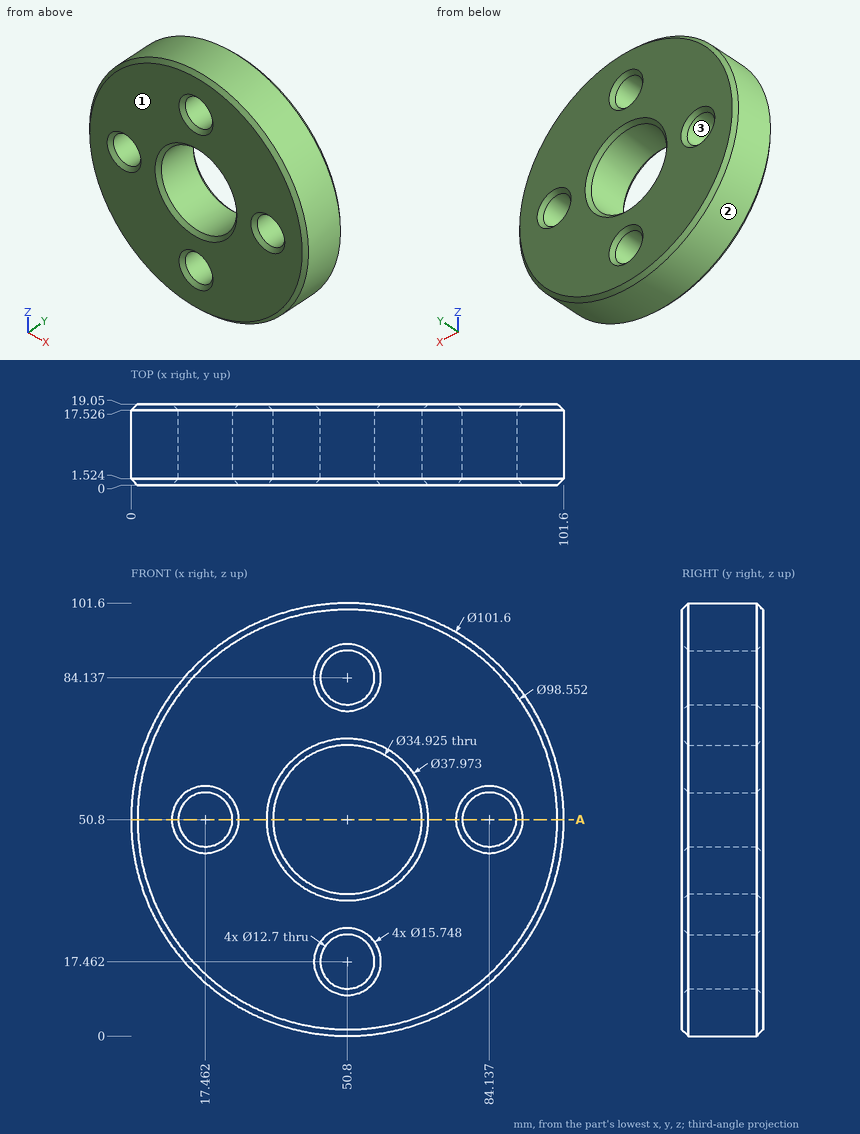
Job drawing, mm, ordinate dimensions from the low corner. One solid piece. Round coordinates to 2 decimals unless told otherwise and drop trailing zeros.
Item 1: Drop flat-ended pins along their axis: P1, Ø10, axis at x = 84.14, z = 50.8, coming from the +Y side; P2, Ø2, axis at x = 26.5, y = 12.5, coming from the -Z side; P3, Ø6, axis at x = 13.5, y = 4, coming from the -Z side; P4, Ø5, axis at x = 16.5, y = 14, coming from the -Z side (1 decimal). Give the stop position or say it passes through.
Item 2: Drill centre lines: line 1 (Z direction, x = 50, y = 2.75) (1 decimal); line 2 (X direction, y = 3.25, z = 53) (1 decimal); line 3 (X direction, y = 6.25, z = 53.5) (1 decimal). Where is each one in solid material? Low to high.
Item 3: Mould opens along Z. For the marked faces 1, 2 and 3 say: +Z half, -Z half, draft (parallel to the pull), parting line (faces both ways), or undercut.
Item 4: Cut at A-A, the plane z = 50.8. State how many separate pieces and enclosed holes the cut face has.
A:
1. P1: passes through
1. P2: stops at z = 5.66
1. P3: stops at z = 13.33
1. P4: stops at z = 11.2
2. line 1: z = 0 to 11.2, 23.8 to 33.4, 68.2 to 77.8, 90.4 to 101.6
2. line 2: x = 0 to 11.5, 23.4 to 33.5, 68.1 to 78.2, 90.1 to 101.6
2. line 3: x = 0.1 to 11.7, 23.2 to 33.5, 68.1 to 78.4, 89.9 to 101.5
3. face 1: draft
3. face 2: parting line
3. face 3: undercut
4. separate pieces: 4
4. enclosed holes: 0
